```python
from build123d import *

# Parameters (mm, degrees)
SKETCH1_R           = 3.175
SKETCH1_R_2         = 9.525
SKETCH1_R_3         = 2.6035
BOSS_EXTRUDE1_DEPTH = 9.525
SKETCH2_R           = 2.6035
CUT_EXTRUDE1_DEPTH  = 12.7


with BuildPart() as part:
    # Sketch1 → Boss-Extrude1 (new body)
    with BuildSketch(Plane.XY.offset(200.726675)):
        with BuildLine():
            Line((-37.090603219, 784.981140976), (-38.887083386, 784.981140976))
            Line((-38.887083386, 784.981140976), (-38.887083386, 740.531140976))
            Line((-38.887083386, 740.531140976), (-37.090603219, 740.531140976))
            ThreePointArc((-37.090603219, 740.531140976), (-34.929955448, 740.01281433), (-33.23961584, 738.570658545))
            ThreePointArc((-33.23961584, 738.570658545), (0, 721.648846957), (33.23961584, 738.570658545))
            ThreePointArc((33.23961584, 738.570658545), (34.929955448, 740.01281433), (37.090603219, 740.531140976))
            Line((37.090603219, 740.531140976), (38.887083386, 740.531140976))
            Line((38.887083386, 740.531140976), (38.887083386, 784.981140976))
            Line((38.887083386, 784.981140976), (37.090603219, 784.981140976))
            ThreePointArc((37.090603219, 784.981140976), (34.929955448, 785.499467621), (33.23961584, 786.941623406))
            ThreePointArc((33.23961584, 786.941623406), (0, 803.863434995), (-33.23961584, 786.941623406))
            ThreePointArc((-33.23961584, 786.941623406), (-34.929955448, 785.499467621), (-37.090603219, 784.981140976))
        make_face()
        with Locations(Location((14.2875, 762.756140976, 0), (0, 0, 180))):
            Circle(SKETCH1_R, mode=Mode.SUBTRACT)
        with Locations(Location((-14.2875, 762.756140976, 0), (0, 0, 180))):
            Circle(SKETCH1_R, mode=Mode.SUBTRACT)
        with Locations(Location((0, 762.756140976, 0), (0, 0, 180))):
            Circle(SKETCH1_R_2, mode=Mode.SUBTRACT)
        with Locations(Location((0, 788.156140976, 0), (0, 0, 180))):
            Circle(SKETCH1_R_3, mode=Mode.SUBTRACT)
        with Locations(Location((-21.997045256, 775.456140976, 0), (0, 0, 180))):
            Circle(SKETCH1_R_3, mode=Mode.SUBTRACT)
        with Locations(Location((-21.997045256, 750.056140976, 0), (0, 0, 180))):
            Circle(SKETCH1_R_3, mode=Mode.SUBTRACT)
        with Locations(Location((0, 737.356140976, 0), (0, 0, 180))):
            Circle(SKETCH1_R_3, mode=Mode.SUBTRACT)
        with Locations(Location((21.997045256, 750.056140976, 0), (0, 0, 180))):
            Circle(SKETCH1_R_3, mode=Mode.SUBTRACT)
        with Locations(Location((21.997045256, 775.456140976, 0), (0, 0, 180))):
            Circle(SKETCH1_R_3, mode=Mode.SUBTRACT)
    extrude(amount=BOSS_EXTRUDE1_DEPTH)

    # Sketch2 → Cut-Extrude1 (cut)
    with BuildSketch(Plane.ZY.offset(38.887083386)):
        with Locations(Location((205.489175, 780.218640976, 0), (0, 0, 270))):
            Circle(SKETCH2_R)
        with Locations(Location((205.489175, 745.293640976, 0), (0, 0, 90))):
            Circle(SKETCH2_R)
    cut_extrude1 = extrude(amount=-CUT_EXTRUDE1_DEPTH, mode=Mode.SUBTRACT)

    # Mirror1: Cut-Extrude1 across plane
    add(cut_extrude1.mirror(Plane(origin=(0, 0, 0), x_dir=(0, 0, 1), z_dir=(1, 0, 0))), mode=Mode.SUBTRACT)


solid = part.part
```
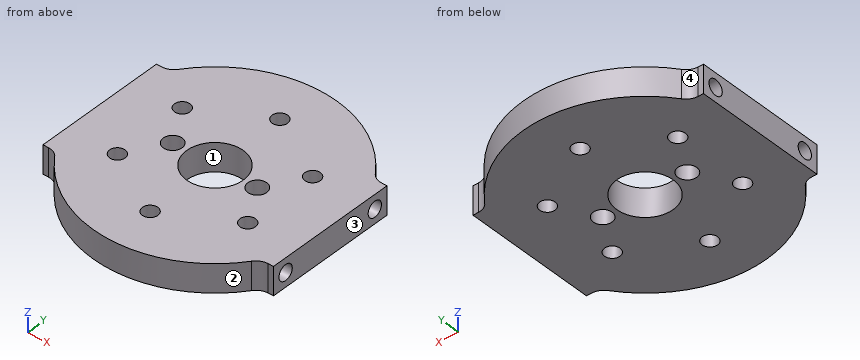
Work out the finished part from the listing and answer in its coordinate system (mm). Face numbers are marked on the shaded views. Round coordinates to 2 decimals unless told otherwise and drop trailing zeros. Loops run counter-clockwise (first coordinate to the right, second up) from the corner with the lowest first, then second, coordinate; pieces in that order, holes last. Notation, with made-up numbers: M 71.25,29 L 122.25,29 A21 ccw 122.25,40 Z; hole C 11,10.25 d11. An arc over 180 degrees is marked long. One line per question, with ' | ' between items.
Q1. Find section A-A, the plane x = 0. Give the vertices of the cut face in (y, z), then the cut area to 3 significant figures.
Conclusion:
outline: M 721.65,200.73 L 734.75,200.73 L 734.75,210.25 L 721.65,210.25 Z; M 739.96,200.73 L 753.23,200.73 L 753.23,210.25 L 739.96,210.25 Z; M 772.28,200.73 L 785.55,200.73 L 785.55,210.25 L 772.28,210.25 Z; M 790.76,200.73 L 803.86,200.73 L 803.86,210.25 L 790.76,210.25 Z | area: 502 mm2
Q2. Each of these flat-tipped pins is pushed along its axis until it touches: pin 1 Ø4.5 at (x, y) = (-22, 775.46) entering from +Z; pin 2 Ø0.9 at (x, z) = (-38, 204.5) entering from -Y; pin 3 Ø3 at (y, z) = (780.22, 205.49) entering from -X; pin 4 Ø1 at (x, z) = (16.5, 208.5) entering from +Y. Where does it stop, or does it pass through?
Conclusion:
pin 1: passes through | pin 2: stops at y = 740.53 | pin 3: stops at x = -26.19 | pin 4: stops at y = 800.62
Q3. The mould has two halves that part along Y. Classify the marked faces 1, 2, 3 and 4: +Y half, -Y half, draft (parallel to the pull), parting line (faces both ways), or undercut.
Conclusion:
face 1: undercut | face 2: -Y half | face 3: draft | face 4: +Y half
Q4. Find section B-B, the plane x = 16.5. Give the vertices of the cut face in (y, z), then the cut area to 3 significant figures.
Conclusion:
outline: M 725.11,200.73 L 760.48,200.73 L 760.48,210.25 L 725.11,210.25 Z; M 765.03,200.73 L 800.41,200.73 L 800.41,210.25 L 765.03,210.25 Z | area: 674 mm2
Q5. Find section D-D, the plane y = 798. Give the vertices of the cut face in (x, z), then the cut area to 3 significant figures.
Conclusion:
outline: M -21.16,200.73 L 21.16,200.73 L 21.16,210.25 L -21.16,210.25 Z | area: 403 mm2
Q6. Consider line 1 along Y through (x, z) = (-0.5, 203); line 2 along Y through (x, z) = (-32, 204.5); line 3 along X through (y, z) = (749, 204.75). Determine where each line is inside the solid, lowest interval first. Write a range as from..to.
Conclusion:
line 1: y = 721.65..734.8, 739.91..753.24, 772.27..785.6, 790.71..803.86 | line 2: y = 736.95..742.89, 747.7..777.81, 782.63..788.56 | line 3: x = -38.89..-24.38, -19.62..19.62, 24.38..38.89
Q7. Find section C-C, the plane z = 204.25. State how many separate pieces and enclosed holes the cut face has, then the cut area to 3 significant figures.
Conclusion:
separate pieces: 1 | enclosed holes: 9 | area: 4,590 mm2
